```python
from build123d import *

# Parameters (mm, degrees)
F1_DEPTH = 7.7
F2_R     = 1.05
F3_DEPTH = 10


# Not quite as in the source:
# - ends of sketch curves that miss each other by under 0.0002 mm in the source are joined


with BuildPart() as f1:
    # F0 (on Top) → F1 (new body)
    with BuildSketch(Plane.XY):
        Polygon((3.85, 0), (0, 0), (-3.85, 0), (-3.85, -12), (-1.35, -12), (-1.35, -5), (0, -5), (1.35, -5), (1.35, -12), (3.85, -12), align=None)
    extrude(amount=F1_DEPTH)

    # F2 (on face) → F3 (cut)
    with BuildSketch(Plane(origin=(-3.85, 0, 0), x_dir=(0, -1, 0), z_dir=(-1, 0, 0))):
        with Locations((8.15, 3.85)):
            Circle(F2_R)
        with BuildLine():
            ThreePointArc((8.3927668004, 7.7), (10.9570802224, 6.4904376141), (12.0000020258, 3.8539515808))
            Line((12.0000020258, 3.8539515808), (12, 7.7))
            Line((12, 7.7), (8.3927668004, 7.7))
        make_face()
        with BuildLine():
            ThreePointArc((12.0000020258, 3.8539515808), (10.8726018857, 1.1301923043), (8.15, 0))
            Line((8.15, 0), (12, 0))
            Line((12, 0), (12.0000020258, 3.8539515808))
        make_face()
    extrude(amount=-F3_DEPTH, mode=Mode.SUBTRACT)


solid = f1.part
```
Here's how the part is built. I have some questions about the finished solid (model axes, mm). A direction names the side the tool comes from. Give positions to 0.01 mm unless a question says otherwise; leave off trailing zeros. Write each loop counter-clockwise with the first axis right and the second up, starting at its lowest first coordinate (ties: lowest second). Pieces come first, ordered by that corner, then holes.
(1) Imagine slicing it at A-A, the plane y = -6.5. Write out the boundary of the cut face in (x, z), and give its area (3 significant figures).
Output values:
outline: (-3.85, 0) - (-1.35, 0) - (-1.35, 7.7) - (-3.85, 7.7) - close; (1.35, 0) - (3.85, 0) - (3.85, 7.7) - (1.35, 7.7) - close
area: 38.5 mm2
(2) Thinking about a two-plate mould opening in X: for faces 1 (the face through (-3.85, -6, 4)), 2 (the face through (1.35, -9, 5)), 3 (the face through (-1.35, -9, 3)), 4 (the face through (2.58, -10.93, 6.52)), which applies, pulls with the +X half, pulls with the -X half, needs draft (parallel to the pull), parting line crosses it, or undercut?
Output values:
face 1: pulls with the -X half
face 2: undercut
face 3: undercut
face 4: needs draft
(3) On a 3-axis mill with a long thin cutter (end or side, diameter ignored), from which of +Z, -Z, +X, -X, +Y, -Y can I reach the whole of each face in a straight line? I mean faces 5 (the face through (-2.62, -10.9, 1.16)), 6 (the face through (0, -5, 4)). Say none if no direction works.
Output values:
face 5: -Z, +X, -X, -Y
face 6: +Z, -Z, -Y
(4) Imagine slicing it at C-C, the plane z = 1.25. Write out the boundary of the cut face in (x, y).
Output values:
outline: (-3.85, -10.99) - (-1.35, -10.99) - (-1.35, -5) - (1.35, -5) - (1.35, -10.99) - (3.85, -10.99) - (3.85, 0) - (-3.85, 0) - close
(5) Imagine slicing it at D-D, the plane y = -9. Write out the boundary of the cut face in (x, z), and give its area (3 significant figures).
Output values:
outline: (-3.85, 0.1) - (-1.35, 0.1) - (-1.35, 3.23) - (-3.85, 3.23) - close; (-3.85, 4.47) - (-1.35, 4.47) - (-1.35, 7.61) - (-3.85, 7.61) - close; (1.35, 0.1) - (3.85, 0.1) - (3.85, 3.23) - (1.35, 3.23) - close; (1.35, 4.47) - (3.85, 4.47) - (3.85, 7.61) - (1.35, 7.61) - close
area: 31.4 mm2
(6) Will these pins go through, and if not, where does the flat tip stop? pin 1 (1.3 mm diameter, centred on y = -8.15, z = 3.85, fed in from -X); pin 2 (2 mm diameter, centred on x = -0.5, z = 3, fed in from -Y).
Output values:
pin 1: passes through
pin 2: stops at y = -11.99
(7) If I drill on L1, parallel to X at y = -8.5, z = 1.25; L2, parallel to Z at x = 2.8, y = -8.15; L3, parallel to Y at x = -0.75, z = 6, over which ranges is the centre line in solid material (lowest first)?
Output values:
L1: x = -3.85 to -1.35, 1.35 to 3.85
L2: z = 0 to 2.8, 4.9 to 7.7
L3: y = -5 to 0
